Design review of the part built by this model. Coordinates are the model's own, in mm. Face numbers are marked on the shaded views. A direction names the side the tool comes from. Coordinates: 2 decimals unless noted, no trailing zeros. Loops run counter-clockwise (first coordinate to the right, second up) from the corner with the lowest first, then second, coordinate; pieces in that order, holes last. Notation, with made-up numbers: M -4,49.5 L 5,49.5 A19 cw 5,78.5 Z; hole C 6.25,-8 d11. An arc over 180 degrees is marked long. Answer as a JSON object with one key per item and string values. Group by question number.
1. Insertion check: pin 1 (1.3 mm diameter, centred on x = 67.9, z = -2.83, fed in from +Y); pin 2 (1.8 mm diameter, centred on x = 68.85, z = 11.81, fed in from +Y); pin 3 (12.5 mm diameter, centred on x = 92, z = 7.5, fed in from -Y) (3 decimals). Each pin has a flat end and moves straight along its axis. Give the tip position at first contact, or say it passes through.
2. To check wall thickness, follow probe 1 along X at (y, z) = (1, -6.5); probe 2 along Y at (x, z) = (67, 9.75) (3 decimals); probe 3 along Y at (x, z) = (111.5, 8.75) (3 decimals). State the ranges of each line that lie inside material, in increasing order.
3. Machinability: for the marked faces 1, 2 and 3, which of the approach directions +Z, -Z, +X, -X, +Y, -Y give a long, thin tool a straight path to every point of the face, cutting with its end or side? Answer none if there is none.
4. Consider section C-C (x = 29.5). State the section outline as (y, z) points (3 decimals), then the cut area to 3 significant figures.
5. Draft analysis for pull direction X (two halves, no side actions). For the marked faces 4, 5 and 6, state which applies: +X half, -X half, draft (parallel to the pull), parting line (faces both ways), or undercut.
6. Consider section B-B (z = 10). State the section outline as (x, y) points (3 decimals), then the cut area to 3 significant figures.
7. Consider section A-A (y = 12). State the section outline as (x, z) points, then the cut area to 3 significant figures.
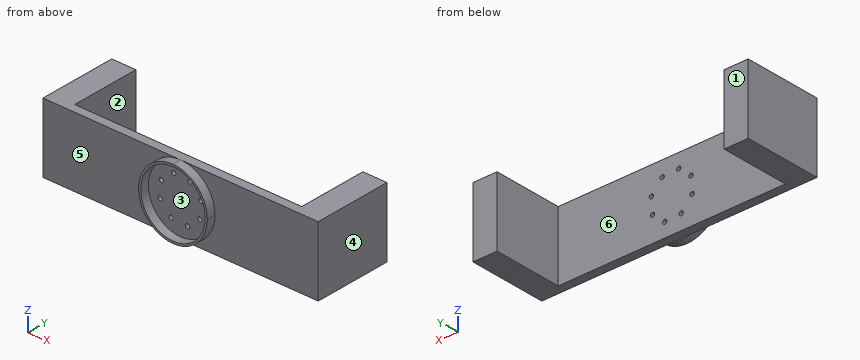
from build123d import *

# Parameters (mm, degrees)
F0_W     = 101.6
F0_H     = 25.4
F1_DEPTH = 3.175
F2_W     = 8.89
F2_H     = 25.4
F3_DEPTH = 25.4
F4_DEPTH = 25.4
F5_R     = 11.90625
F6_DEPTH = 3.175
F7_R     = 0.79375
F8_DEPTH = 25.4


with BuildPart() as f1:
    # F0 (on Front) → F1 (new body)
    with BuildSketch(Plane.XZ):
        with Locations((65.346594, 4.688971)):
            Rectangle(F0_W, F0_H)
    extrude(amount=F1_DEPTH)

    # F2 (on face) → F3 (join)
    with BuildSketch(Plane(origin=(0, 0, 0), x_dir=(-1, 0, 0), z_dir=(0, 1, 0))):
        with Locations((-111.701594, 4.688971)):
            Rectangle(F2_W, F2_H)
    extrude(amount=F3_DEPTH)

    # F2 (on face) → F4 (join)
    with BuildSketch(Plane(origin=(0, 0, 0), x_dir=(-1, 0, 0), z_dir=(0, 1, 0))):
        with Locations((-18.991594, 4.688971)):
            Rectangle(F2_W, F2_H)
    extrude(amount=F4_DEPTH)

    # F5 (on face) → F6 (join)
    with BuildSketch(Plane.XZ.offset(3.175)):
        with BuildLine():
            ThreePointArc((65.346594, -8.011029), (74.32685, -4.291285), (78.046594, 4.688971))
            ThreePointArc((78.046594, 4.688971), (74.32685, 13.669228), (65.346594, 17.388971))
            ThreePointArc((65.346594, 17.388971), (52.646594, 4.688971), (65.346594, -8.011029))
        make_face()
        with Locations((65.346594, 4.688971)):
            Circle(F5_R, mode=Mode.SUBTRACT)
    extrude(amount=F6_DEPTH)

    # F7 (on face) → F8 (cut)
    with BuildSketch(Plane.XZ.offset(3.175)):
        with Locations((58.226489, 8.197249)):
            Circle(F7_R)
        with Locations((62.792646, 12.204373)):
            Circle(F7_R)
        with Locations((68.854871, 11.809077)):
            Circle(F7_R)
        with Locations((72.861995, 7.242919)):
            Circle(F7_R)
        with Locations((72.466699, 1.180694)):
            Circle(F7_R)
        with Locations((67.900542, -2.82643)):
            Circle(F7_R)
        with Locations((61.838316, -2.431134)):
            Circle(F7_R)
        with Locations((57.831193, 2.135024)):
            Circle(F7_R)
    extrude(amount=-F8_DEPTH, mode=Mode.SUBTRACT)


solid = f1.part
Findings below:
{
 "1": {"pin 1": "passes through", "pin 2": "stops at y = 0", "pin 3": "stops at y = -3.175"},
 "2": {"probe 1": "x = 14.55 to 23.44, 107.26 to 116.15", "probe 2": "y = -3.175 to 0", "probe 3": "y = -3.175 to 25.4"},
 "3": {"face 1": "+Z, -Z, +X, -X, +Y", "face 2": "+Z, -Z, +Y", "face 3": "-Y"},
 "4": {"outline": "M -3.175,-8.011 L 0,-8.011 L 0,17.389 L -3.175,17.389 Z", "area": "80.6 mm^2"},
 "5": {"face 4": "+X half", "face 5": "draft", "face 6": "undercut"},
 "6": {"outline": "M 14.547,-3.175 L 53.81,-3.175 L 53.81,-6.35 L 54.691,-6.35 L 54.691,-3.175 L 76.003,-3.175 L 76.003,-6.35 L 76.883,-6.35 L 76.883,-3.175 L 116.147,-3.175 L 116.147,25.4 L 107.257,25.4 L 107.257,0 L 23.437,0 L 23.437,25.4 L 14.547,25.4 Z", "area": "780 mm^2"},
 "7": {"outline": "M 14.55,-8.01 L 23.44,-8.01 L 23.44,17.39 L 14.55,17.39 Z; M 107.26,-8.01 L 116.15,-8.01 L 116.15,17.39 L 107.26,17.39 Z", "area": "452 mm^2"}
}
